The model under review builds one solid part; all positions refer to its coordinate system, in mm. A direction names the side the tool comes from. Coordinates: 2 decimals unless noted, no trailing zeros. Write each loop counter-clockwise with the first axis right and the second up, starting at its lowest first coordinate (ties: lowest second). Pieces come first, ordered by that corner, then holes.
```python
from build123d import *

# Parameters (mm, degrees)
SKETCH006_R  = 1.4
PAD004_DEPTH = 7.5
PAD005_DEPTH = 1
PAD_DEPTH    = 1
PAD006_DEPTH = 27


with BuildPart() as mount:
    # Sketch006 → Pad004 (new body)
    with BuildSketch(Plane.XZ):
        with Locations((-15, 13.5)):
            Circle(SKETCH006_R)
        with Locations((15, 13.5)):
            Circle(SKETCH006_R)
    extrude(amount=-PAD004_DEPTH)


with BuildPart() as toplip:
    # Sketch005 → Pad005 (new body)
    with BuildSketch(Plane.XY.offset(26)):
        with BuildLine():
            ThreePointArc((7.46, 0), (0, 7.46), (-7.46, 0))
            Line((-7.46, 0), (-6, 0))
            ThreePointArc((6, 0), (0, 6), (-6, 0))
            Line((7.46, 0), (6, 0))
        make_face()
    extrude(amount=PAD005_DEPTH)


with BuildPart() as bottomlip:
    # Sketch003 → Pad (new body)
    with BuildSketch(Plane.XY):
        with BuildLine():
            ThreePointArc((7.46, 0), (0, 7.46), (-7.46, 0))
            Line((-7.46, 0), (-6, 0))
            ThreePointArc((6, 0), (0, 6), (-6, 0))
            Line((7.46, 0), (6, 0))
        make_face()
    extrude(amount=PAD_DEPTH)


with BuildPart() as final:
    # Sketch → Pad006 (new body)
    with BuildSketch(Plane.XY):
        with BuildLine():
            ThreePointArc((7.45, 0), (0, 7.45), (-7.45, 0))
            Line((-7.45, 0), (-21.8427, 0))
            Line((-21.8427, 0), (-21.8427, 7.5))
            Line((-21.8427, 7.5), (21.8427, 7.5))
            Line((21.8427, 0), (21.8427, 7.5))
            Line((7.45, 0), (21.8427, 0))
        make_face()
    extrude(amount=PAD006_DEPTH)

    # Fusion: union TopLip, BottomLip
    add(toplip.part)
    add(bottomlip.part)

    # Cut: cut Mount
    add(mount.part, mode=Mode.SUBTRACT)


solid = final.part
```
Item 1: Take a section at B-B, the plane y = 2.75. Write out the cut boundary in (x, z).
Solved:
outline: (-21.84, 0) - (-5.33, 0) - (-5.33, 1) - (-6.92, 1) - (-6.92, 26) - (-5.33, 26) - (-5.33, 27) - (-21.84, 27) - close; (5.33, 0) - (21.84, 0) - (21.84, 27) - (5.33, 27) - (5.33, 26) - (6.92, 26) - (6.92, 1) - (5.33, 1) - close; hole circle Ø2.8 at (-15, 13.5); hole circle Ø2.8 at (15, 13.5)
Item 2: Take a section at C-C, the plane x = -15. Write out the cut boundary in (y, z), plus the area to 4 significant figures.
Solved:
outline: (0, 0) - (7.5, 0) - (7.5, 12.1) - (0, 12.1) - close; (0, 14.9) - (7.5, 14.9) - (7.5, 27) - (0, 27) - close
area: 181.5 mm2
Item 3: Machinability: for faces 4 (the face through (-2.393, 7.055, 13.325)), 5 (the face through (12, 0, 13)), which of the approach directions +Z, -Z, +X, -X, +Y, -Y give a long, thin tool a straight path to every point of the face, cutting with its end or side? Answer none if there is none.
Solved:
face 4: -Y
face 5: +Z, -Z, +X, -X, -Y
Item 4: Take a section at A-A, the plane z = 13.5. Write out the cut boundary in (x, y).
Solved:
outline: (-21.84, 0) - (-16.4, 0) - (-16.4, 7.5) - (-21.84, 7.5) - close; (-13.6, 0) - (-7.45, 0) arc R7.45 cw to (7.45, 0) - (13.6, 0) - (13.6, 7.5) - (-13.6, 7.5) - close; (16.4, 0) - (21.84, 0) - (21.84, 7.5) - (16.4, 7.5) - close
Item 5: For pin 1 (3 mm diameter, centred on x = -15, z = 13.5, fed in from +Y), flat-tipped, find the tip position at first contact; note if it passes through.
Solved:
pin 1: stops at y = 7.5
Item 6: Mouldability with a two-part tool opening along X and no side actions: class faces 1 (the face through (0.3, 6.3, 0)), 2 (the face through (0.5, 6.2, 1)), 3 (the face through (21.843, 4, 13)) as pulls with the +X half, pulls with the -X half, needs draft (parallel to the pull), parting line crosses it, or undercut.
Solved:
face 1: needs draft
face 2: undercut
face 3: pulls with the +X half
Item 7: To check wall thickness, follow line 1 along Z through (x, y) = (15, 2.5); line 2 along X through (y, z) = (2.5, 19.5); line 3 along X through (y, z) = (4.5, 24.5). State the ranges of each line that lie inside material, in increasing order.
Solved:
line 1: z = 0 to 12.1, 14.9 to 27
line 2: x = -21.84 to -7.02, 7.02 to 21.84
line 3: x = -21.84 to -5.94, 5.94 to 21.84
